Design review of the part built by this model. Coordinates are the model's own, in mm. Coordinates: 2 decimals unless noted, no trailing zeros. Write each loop counter-clockwise with the first axis right and the second up, starting at its lowest first coordinate (ties: lowest second). Pieces come first, ordered by that corner, then holes.
Q1. Add section B-B, the plane x = 6.5. Give the boundary of the cut face in (y, z) (3 decimals).
Q2. Clearance check with flat-ended pins moving along their axes: pin 1 Ø12 at (x, z) = (65.5, 17) entering from +Y; pin 2 Ø2.5 at (x, y) = (13, 1.5) entering from +Z; pin 3 Ø1 at (x, y) = (6.5, -1) entering from +Z. State where each tip first meets the part, or that it passes through.
Q3. Add section C-C, the plane z = -21.5. Give the boundary of the cut face in (x, y) (3 decimals), plus the area to 3 significant figures.
Q4. Add section A-A, the plane y = 1.25. Give the boundary of the cut face in (x, z).
Q5. To check wall thickness, follow probe 1 along Y at (x, z) = (61.5, -10) (3 decimals); probe 2 along X at (y, z) = (1, -30.5); probe 3 along Z at (x, y) = (58.5, -0.5). State the ranges of each line that lie inside material, in increasing order.
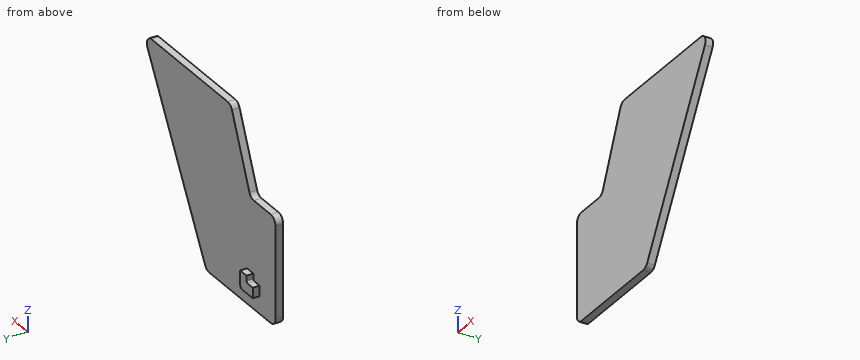
from build123d import *

# Parameters (mm, degrees)
EXTRUDE1_DEPTH = 3.175
EXTRUDE2_DEPTH = 2.8575


with BuildPart() as part:
    # Sketch1 → Extrude1 (new body)
    with BuildSketch(Plane(origin=(0, 0, 0), x_dir=(1, 0, 0), z_dir=(0, 1, 0))):
        with BuildLine():
            Line((3.175, 44.50785877), (45.047498502, 44.50785877))
            ThreePointArc((45.047498502, 44.50785877), (46.651643951, 44.072811758), (47.81618078, 42.886893339))
            Line((47.81618078, 42.886893339), (87.038547596, -26.992036046))
            ThreePointArc((87.038547596, -26.992036046), (87.009818306, -30.150216064), (84.269865318, -31.721070615))
            Line((84.269865318, -31.721070615), (32.528914715, -31.721070615))
            ThreePointArc((32.528914715, -31.721070615), (30.778624678, -31.195053398), (29.608292243, -29.791297251))
            Line((29.608292243, -29.791297251), (17.72934795, -1.929773364))
            ThreePointArc((17.72934795, -1.929773364), (16.559015516, -0.526017217), (14.808725478, 0))
            Line((14.808725478, 0), (3.175, 0))
            ThreePointArc((3.175, 0), (0.92993597, 0.92993597), (0, 3.175))
            Line((0, 3.175), (0, 41.33285877))
            ThreePointArc((0, 41.33285877), (0.92993597, 43.5779228), (3.175, 44.50785877))
        make_face()
    extrude(amount=-EXTRUDE1_DEPTH)

    # Sketch4 → Extrude2 (add, symmetric)
    with BuildSketch(Plane(origin=(0, 0, 0), x_dir=(1, 0, 0), z_dir=(0, 1, 0))):
        with BuildLine():
            Line((10.768757098, 37.225043705), (17.854525476, 37.225043705))
            ThreePointArc((17.854525476, 37.225043705), (18.93215621, 36.77867444), (19.378525476, 35.701043705))
            Line((19.378525476, 35.701043705), (19.378525476, 30.0552377))
            Line((19.378525476, 30.0552377), (15.061814646, 30.0552377))
            Line((15.061814646, 30.0552377), (15.061814646, 32.146332876))
            ThreePointArc((15.061814646, 32.146332876), (14.838630013, 32.685148243), (14.299814646, 32.908332876))
            Line((14.299814646, 32.908332876), (10.768757098, 32.908332876))
            Line((10.768757098, 32.908332876), (10.768757098, 37.225043705))
        make_face()
    extrude(amount=EXTRUDE2_DEPTH, both=True)


solid = part.part
Here are the results:
1. outline: (-3.175, -44.508) - (0, -44.508) - (0, 0) - (-3.175, 0) - close
2. pin 1: stops at y = 0
2. pin 2: stops at z = -32.91
2. pin 3: stops at z = 0
3. outline: (0, -3.175) - (59.82, -3.175) - (59.82, 0) - (0, 0) - close
3. area: 190 mm2
4. outline: (10.77, -37.23) - (17.85, -37.23) arc R1.52 ccw to (19.38, -35.7) - (19.38, -30.06) - (15.06, -30.06) - (15.06, -32.15) arc R0.76 cw to (14.3, -32.91) - (10.77, -32.91) - close
5. probe 1: y = -3.175 to 0
5. probe 2: x = 15.06 to 19.38
5. probe 3: z = -23.85 to 31.72
